For this review, take the finished solid that the model builds, in its own axes (mm). A direction names the side the tool comes from. Give positions to 0.01 mm unless a question says otherwise; leave off trailing zeros. Write each loop counter-clockwise with the first axis right and the second up, starting at its lowest first coordinate (ties: lowest second). Pieces come first, ordered by that corner, then holes. Notation, with made-up numbers: M 83.5,-36.75 L 105.5,-36.75 A29 ccw 105.5,-3.75 Z; hole C 30,-39.75 d6. An arc over 180 degrees is marked long. Answer as a JSON object with one key per item and string values. Group by question number.
```python
from build123d import *

# Parameters (mm, degrees)
F0_W     = 27.94
F0_H     = 22.86
F0_W_2   = 15.24
F0_H_2   = 10.16
F1_DEPTH = 1.5875
F2_R     = 2.54
F2_R_2   = 1.016
F3_DEPTH = 3.175
F4_DEPTH = 25.4


with BuildPart() as f1:
    # F0 (on Top) → F1 (new body)
    with BuildSketch(Plane.XY):
        Rectangle(F0_W, F0_H)
        Rectangle(F0_W_2, F0_H_2, mode=Mode.SUBTRACT)
    extrude(amount=F1_DEPTH)

    # F2 (on face) → F3 (join)
    with BuildSketch(Plane.XY.offset(1.5875)):
        with Locations((-10.795, -7.62)):
            Circle(F2_R)
        with Locations((-10.795, -7.62)):
            Circle(F2_R_2, mode=Mode.SUBTRACT)
        with Locations((-10.795, 7.62)):
            Circle(F2_R)
        with Locations((-10.795, 7.62)):
            Circle(F2_R_2, mode=Mode.SUBTRACT)
        with Locations((10.795, -7.62)):
            Circle(F2_R)
        with Locations((10.795, -7.62)):
            Circle(F2_R_2, mode=Mode.SUBTRACT)
        with Locations((10.795, 7.62)):
            Circle(F2_R)
        with Locations((10.795, 7.62)):
            Circle(F2_R_2, mode=Mode.SUBTRACT)
    extrude(amount=F3_DEPTH)

    # F2 (on face) → F4 (cut)
    with BuildSketch(Plane.XY.offset(1.5875)):
        with Locations((10.795, -7.62)):
            Circle(F2_R_2)
        with Locations((10.795, 7.62)):
            Circle(F2_R_2)
        with Locations((-10.795, 7.62)):
            Circle(F2_R_2)
        with Locations((-10.795, -7.62)):
            Circle(F2_R_2)
    extrude(amount=-F4_DEPTH, mode=Mode.SUBTRACT)


solid = f1.part
```
Item 1: Draft analysis for pull direction X (two halves, no side actions). For faces 1 (the flat face through (0, -5.08, 1)), 2 (the flat face through (-13.97, 0, 1)), 3 (the cylindrical face through (-8.37, -6.86, 3.15)), 4 (the flat face through (-11, -9, 4.762)), state which applies: released by +X, released by -X, zero draft, split by the parting line, or undercut.
Item 2: Consider section C-C (y = 0). Give the boundary of the cut face in (x, z).
Item 3: Insertion check: P1, Ø1.8, axis at x = -10.795, y = 7.62, coming from the +Z side; P2, Ø1.5, axis at x = 9.5, z = 3, coming from the -Y side; P3, Ø1, axis at y = 7.5, z = 2.5, coming from the -X side (3 decimals); P4, Ø4, axis at x = -8, y = -1, coming from the +Z side. Each pin has a flat end and moves straight along its axis. Give the tip position at first contact, or say it passes through.
Item 4: To check wall thickness, follow probe 1 along Z at (x, y) = (-11, -0.5); probe 2 along X at (y, z) = (-9, 2.95); probe 3 along Y at (x, z) = (-9.5, 4.35). State the ranges of each line that lie inside material, in increasing order.
Item 5: Consider section D-D (y = 7.62). Give the boundary of the cut face in (x, z) (1 decimal).
Item 6: Machinability: for faces 5 (the flat face through (-0.2, 5.24, 1.588)), 6 (the flat face through (-0.2, 5.24, 0)), 7 (the flat face through (0, 5.08, 1)), which of the approach directions +Z, -Z, +X, -X, +Y, -Y give a long, thin tool a straight path to every point of the face, cutting with its end or side? Answer none if there is none.
Item 7: Consider section B-B (z = 3.45). Give the boundary of the cut face in (x, y) (3 decimals), plus the area to 3 significant figures.
Item 8: Consider section A-A (x = -4.5). Give the boundary of the cut face in (y, z), plus the area to 3 significant figures.
Result set:
{
 "1": {"face 1": "undercut", "face 2": "released by -X", "face 3": "undercut", "face 4": "zero draft"},
 "2": {"outline": "M -13.97,0 L -7.62,0 L -7.62,1.59 L -13.97,1.59 Z; M 7.62,0 L 13.97,0 L 13.97,1.59 L 7.62,1.59 Z"},
 "3": {"P1": "passes through", "P2": "stops at y = -10.1", "P3": "stops at x = -13.335", "P4": "stops at z = 1.59"},
 "4": {"probe 1": "z = 0 to 1.59", "probe 2": "x = -12.93 to -8.66, 8.66 to 12.93", "probe 3": "y = -9.81 to -5.43, 5.43 to 9.81"},
 "5": {"outline": "M -14,0 L -11.8,0 L -11.8,4.8 L -13.3,4.8 L -13.3,1.6 L -14,1.6 Z; M -9.8,0 L 9.8,0 L 9.8,4.8 L 8.3,4.8 L 8.3,1.6 L -8.3,1.6 L -8.3,4.8 L -9.8,4.8 Z; M 11.8,0 L 14,0 L 14,1.6 L 13.3,1.6 L 13.3,4.8 L 11.8,4.8 Z"},
 "6": {"face 5": "+Z", "face 6": "-Z, +X, -X, +Y, -Y", "face 7": "+Z, -Z"},
 "7": {"outline": "C -10.795,-7.62 d5.08; C -10.795,7.62 d5.08; C 10.795,-7.62 d5.08; C 10.795,7.62 d5.08; hole C -10.795,-7.62 d2.032; hole C -10.795,7.62 d2.032; hole C 10.795,-7.62 d2.032; hole C 10.795,7.62 d2.032", "area": "68.1 mm^2"},
 "8": {"outline": "M -11.43,0 L -5.08,0 L -5.08,1.59 L -11.43,1.59 Z; M 5.08,0 L 11.43,0 L 11.43,1.59 L 5.08,1.59 Z", "area": "20.2 mm^2"}
}
